Geometry: final body of the model. Coordinates: model frame, mm. Face numbers are marked on the shaded views. A direction names the side the tool comes from. Give positions to 0.01 mm unless a question says otherwise; leave off trailing zeros. Write each loop counter-clockwise with the first axis right and the second up, starting at its lowest first coordinate (ties: lowest second). Pieces come first, ordered by that corner, then holes. Notation, with made-up numbers: M 4,1 L 46,1 A23 cw 46,14 Z; hole C 80.5,-4 d11. An arc over 180 degrees is marked long. Use a Markdown table: item, result. Add a question column.
(1) Cut plane C-C (z = 36.5). Output: boundary loops of the cut face in (x, y).
(2) Material intervals for L1, parallel to X at y = -5.5, z = 39; L2, parallel to Y at x = 4, z = -24.5; L3, parallel to Z at x = 4.75, y = 32.5, sorted ascending.
(3) Cut plane A-A (x = 8.25). Output: boundary loops of the cut face in (y, z), plus the area to 3 significant figures.
(4) Cut plane D-D (y = -11). Output: boundary loops of the cut face in (x, z).
(5) Pin query (flat end, axial travel): pin 1 Ø13 at (y, z) = (1.5, -23) entering from +X; pin 2 Ø1.5 at (x, y) = (13, -1.5) entering from +Z; pin 3 Ø8 at (x, z) = (13, 29) entering from -Y. Return the tip coordinate at first contact, or that it passes through.
(6) Reachability of the marked faces 1, 2 and 3 from +Z, -Z, +X, -X, +Y, -Y: full face, straight path, thin tool, end or side. Return the list, or none.
(7) Cut plane B-B (y = 0). Output: boundary loops of the cut face in (x, z).
(8) Draft query along Y for the marked faces 4, 5 and 6. Return one class per face: released by +Y, released by -Y, zero draft, split by the parting line, or undercut.
```python
from build123d import *

# Parameters (mm, degrees)
BOSS_EXTRUDE3_DEPTH = 15
SKETCH3_R           = 4
CUT_EXTRUDE3_DEPTH  = 14.0462
CUT_EXTRUDE4_DEPTH  = 3
MIRROR1_START       = 12
MIRROR1_DEPTH       = 3
MIRROR1_2_DEPTH     = 12
MIRROR1_3_DEPTH     = 3


# Read off the part's stored shape, not the designer's step: Mirror1
with BuildPart() as part:
    # Sketch1 → Boss-Extrude3 (new body)
    with BuildSketch(Plane.YZ):
        with BuildLine():
            Line((-28.968617751, -12.789334175), (28.968617751, -12.789334175))
            ThreePointArc((28.968617751, -12.789334175), (44.579120821, 0), (35.110840206, 17.821518929))
            ThreePointArc((35.110840206, 17.821518929), (30.644623053, 21.505675602), (28.968617751, 27.047436358))
            Line((28.968617751, 27.047436358), (28.968617751, 39.053986921))
            ThreePointArc((28.968617751, 39.053986921), (26.039685563, 46.125054733), (18.968617751, 49.053986921))
            Line((18.968617751, 49.053986921), (-18.968617751, 49.053986921))
            ThreePointArc((-18.968617751, 49.053986921), (-26.039685563, 46.125054733), (-28.968617751, 39.053986921))
            Line((-28.968617751, 39.053986921), (-28.968617751, 27.047436358))
            ThreePointArc((-28.968617751, 27.047436358), (-30.644623053, 21.505675602), (-35.110840206, 17.821518929))
            ThreePointArc((-35.110840206, 17.821518929), (-44.579120821, 0), (-28.968617751, -12.789334175))
        make_face()
    extrude(amount=BOSS_EXTRUDE3_DEPTH)

    # Sketch3 → Cut-Extrude3 (cut)
    with BuildSketch(Plane.YZ.offset(15)):
        with Locations(Location((0, 3.132326373, 0), (0, 0, 270))):
            Circle(SKETCH3_R)
    extrude(amount=-CUT_EXTRUDE3_DEPTH, mode=Mode.SUBTRACT)

    # Sketch4 → Cut-Extrude4 (cut)
    with BuildSketch(Plane.YZ.offset(15)):
        with BuildLine():
            Line((-12.95, 49.053986921), (-12.95, 31.267703884))
            ThreePointArc((-12.95, 31.267703884), (0, 18.317703884), (12.95, 31.267703884))
            Line((12.95, 31.267703884), (12.95, 49.053986921))
            Line((12.95, 49.053986921), (-12.95, 49.053986921))
        make_face()
    extrude(amount=-CUT_EXTRUDE4_DEPTH, mode=Mode.SUBTRACT)

    # Mirror1 outline → Mirror1 (cut)
    with BuildSketch(Plane.YZ.offset(MIRROR1_START)):
        with BuildLine():
            ThreePointArc((4.30437196, -12.789334175), (0, -12.053051137), (-4.30437196, -12.789334175))
            Line((-4.30437196, -12.789334175), (4.30437196, -12.789334175))
        make_face()
    extrude(amount=MIRROR1_DEPTH, mode=Mode.SUBTRACT)

    # Mirror1 2 outline → Mirror1 2 (add)
    with BuildSketch(Plane.YZ):
        with BuildLine():
            ThreePointArc((-28.968617751, -32.789334175), (-26.039685563, -39.860401987), (-18.968617751, -42.789334175))
            Line((-18.968617751, -42.789334175), (18.968617751, -42.789334175))
            ThreePointArc((18.968617751, -42.789334175), (26.039685563, -39.860401987), (28.968617751, -32.789334175))
            Line((28.968617751, -32.789334175), (28.968617751, -20.782783611))
            ThreePointArc((28.968617751, -20.782783611), (30.644623053, -15.241022855), (35.110840206, -11.556866182))
            ThreePointArc((35.110840206, -11.556866182), (32.100944124, -12.478176697), (28.968617751, -12.789334175))
            Line((28.968617751, -12.789334175), (-28.968617751, -12.789334175))
            ThreePointArc((-28.968617751, -12.789334175), (-32.100944124, -12.478176697), (-35.110840206, -11.556866182))
            ThreePointArc((-35.110840206, -11.556866182), (-30.644623053, -15.241022855), (-28.968617751, -20.782783611))
            Line((-28.968617751, -20.782783611), (-28.968617751, -32.789334175))
        make_face()
    extrude(amount=MIRROR1_2_DEPTH)

    # Mirror1 3 outline → Mirror1 3 (add)
    with BuildSketch(Plane.YZ.offset(MIRROR1_START)):
        with BuildLine():
            ThreePointArc((-28.968617751, -32.789334175), (-26.039685563, -39.860401987), (-18.968617751, -42.789334175))
            Line((-18.968617751, -42.789334175), (-12.95, -42.789334175))
            Line((-12.95, -42.789334175), (-12.95, -25.003051137))
            ThreePointArc((-12.95, -25.003051137), (-10.569865583, -17.521043281), (-4.30437196, -12.789334175))
            Line((-4.30437196, -12.789334175), (-28.968617751, -12.789334175))
            ThreePointArc((-28.968617751, -12.789334175), (-32.100944124, -12.478176697), (-35.110840206, -11.556866182))
            ThreePointArc((-35.110840206, -11.556866182), (-30.644623053, -15.241022855), (-28.968617751, -20.782783611))
            Line((-28.968617751, -20.782783611), (-28.968617751, -32.789334175))
        make_face()
        with BuildLine():
            Line((12.95, -25.003051137), (12.95, -42.789334175))
            Line((12.95, -42.789334175), (18.968617751, -42.789334175))
            ThreePointArc((18.968617751, -42.789334175), (26.039685563, -39.860401987), (28.968617751, -32.789334175))
            Line((28.968617751, -32.789334175), (28.968617751, -20.782783611))
            ThreePointArc((28.968617751, -20.782783611), (30.644623053, -15.241022855), (35.110840206, -11.556866182))
            ThreePointArc((35.110840206, -11.556866182), (32.100944124, -12.478176697), (28.968617751, -12.789334175))
            Line((28.968617751, -12.789334175), (4.30437196, -12.789334175))
            ThreePointArc((4.30437196, -12.789334175), (10.569865583, -17.521043281), (12.95, -25.003051137))
        make_face()
        with BuildLine():
            ThreePointArc((-4.304371959, 19.053986921), (0, 18.317703884), (4.304371959, 19.053986921))
            Line((4.304371959, 19.053986921), (-4.304371959, 19.053986921))
        make_face()
    extrude(amount=MIRROR1_3_DEPTH)


solid = part.part
```
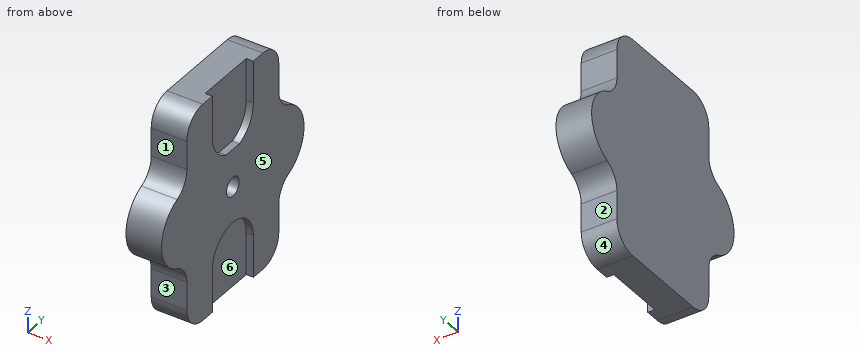
Answer list:
| question | item | result |
|---|---|---|
| 1 | outline | M 0,-28.97 L 15,-28.97 L 15,-12.95 L 12,-12.95 L 12,12.95 L 15,12.95 L 15,28.97 L 0,28.97 Z |
| 2 | L1 | 0 to 12 |
| 2 | L2 | -28.97 to 28.97 |
| 2 | L3 | -13.16 to 19.42 |
| 3 | outline | M -35.11,-11.56 A10 cw -28.97,-20.78 L -28.97,-32.79 A10 ccw -18.97,-42.79 L 18.97,-42.79 A10 ccw 28.97,-32.79 L 28.97,-20.78 A10 cw 35.11,-11.56 A15.92 ccw 35.11,17.82 A10 cw 28.97,27.05 L 28.97,39.05 A10 ccw 18.97,49.05 L -18.97,49.05 A10 ccw -28.97,39.05 L -28.97,27.05 A10 cw -35.11,17.82 A15.92 ccw Z; hole C 0,3.13 d8 |
| 3 | area | 6,020 mm² |
| 4 | outline | M 0,-42.79 L 12,-42.79 L 12,-18.17 L 15,-18.17 L 15,24.43 L 12,24.43 L 12,49.05 L 0,49.05 Z |
| 5 | pin 1 | x = 12 |
| 5 | pin 2 | z = 19.05 |
| 5 | pin 3 | y = -29.18 |
| 6 | face 1 | +Z, +X, -X, -Y |
| 6 | face 2 | -Z, +X, -X, +Y |
| 6 | face 3 | -Z, +X, -X, -Y |
| 7 | outline | M 0,-42.79 L 12,-42.79 L 12,-12.05 L 15,-12.05 L 15,-0.87 L 0.95,-0.87 L 0.95,7.13 L 15,7.13 L 15,19.05 L 12,19.05 L 12,49.05 L 0,49.05 Z |
| 8 | face 4 | released by +Y |
| 8 | face 5 | zero draft |
| 8 | face 6 | undercut |
